Here's how the part is built. I have some questions about the finished solid (model axes, mm). A direction names the side the tool comes from. Round coordinates to 2 decimals unless told otherwise and drop trailing zeros. Order: outer loops, then holes, each group sorted by start corner. A loop starts at its lowest first (then second) coordinate and runs counter-clockwise, first axis right, second up.
```python
from build123d import *

# Parameters (mm, degrees)
SKETCH_1_R          = 14
EXTRUDE_1_DEPTH     = 5
SKETCH_2_R          = 14
EXTRUDE_2_DEPTH     = 5
SKETCH_4_R          = 3.8
EXTRUDE_3_DEPTH     = 25
FILLET_1_R          = 2
SKETCH_3_W          = 3.2
SKETCH_3_H          = 5.5
CUT_EXTRUDE_1_DEPTH = 5.5


with BuildPart() as part:
    # Эскиз1 → Бобышка-Вытянуть1 (new body)
    with BuildSketch(Plane(origin=(0, 0, 0), x_dir=(1, 0, 0), z_dir=(0, 1, 0))):
        with Locations(Location((0, 0, 0), (0, 0, 270))):
            Circle(SKETCH_1_R)
        with BuildLine():
            ThreePointArc((-7.383246629, 9.45979224), (-7.957471899, 8.982128978), (-8.500867665, 8.469666401))
            ThreePointArc((-8.500867665, 8.469666401), (-8.106391079, 5.595437755), (-10.933724873, 4.945064246))
            ThreePointArc((-10.933724873, 4.945064246), (-11.220194912, 4.255258645), (-11.463194733, 3.548966963))
            ThreePointArc((-11.463194733, 3.548966963), (-9.77818241, 1.187286301), (-11.979418514, -0.702518371))
            ThreePointArc((-11.979418514, -0.702518371), (-11.912506489, -1.446440163), (-11.799442035, -2.184758036))
            ThreePointArc((-11.799442035, -2.184758036), (-9.20990999, -3.492858137), (-10.280771741, -6.189162496))
            ThreePointArc((-10.280771741, -6.189162496), (-9.875806391, -6.816776961), (-9.432579364, -7.417981298))
            ThreePointArc((-9.432579364, -7.417981298), (-6.531758184, -7.372830869), (-6.226924059, -10.25794408))
            ThreePointArc((-6.226924059, -10.25794408), (-5.576678065, -10.625472308), (-4.904826437, -10.951834441))
            ThreePointArc((-4.904826437, -10.951834441), (-2.357259293, -9.563776902), (-0.746563118, -11.976754298))
            ThreePointArc((-0.746563118, -11.976754298), (0, -12), (0.746563118, -11.976754298))
            ThreePointArc((0.746563118, -11.976754298), (2.357259293, -9.563776902), (4.904826437, -10.951834441))
            ThreePointArc((4.904826437, -10.951834441), (5.576678065, -10.625472308), (6.226924059, -10.25794408))
            ThreePointArc((6.226924059, -10.25794408), (6.531758184, -7.372830869), (9.432579364, -7.417981298))
            ThreePointArc((9.432579364, -7.417981298), (9.875806391, -6.816776961), (10.280771741, -6.189162496))
            ThreePointArc((10.280771741, -6.189162496), (9.20990999, -3.492858137), (11.799442035, -2.184758036))
            ThreePointArc((11.799442035, -2.184758036), (11.912506489, -1.446440163), (11.979418514, -0.702518371))
            ThreePointArc((11.979418514, -0.702518371), (9.77818241, 1.187286301), (11.463194733, 3.548966963))
            ThreePointArc((11.463194733, 3.548966963), (11.220194912, 4.255258645), (10.933724873, 4.945064246))
            ThreePointArc((10.933724873, 4.945064246), (8.106391079, 5.595437755), (8.500867665, 8.469666401))
            ThreePointArc((8.500867665, 8.469666401), (7.957471899, 8.982128978), (7.383246629, 9.45979224))
            ThreePointArc((7.383246629, 9.45979224), (4.577523245, 8.721741853), (3.591094261, 11.450067336))
            ThreePointArc((3.591094261, 11.450067336), (2.871787971, 11.651301809), (2.14135556, 11.807395833))
            ThreePointArc((2.14135556, 11.807395833), (0, 9.85), (-2.14135556, 11.807395833))
            ThreePointArc((-2.14135556, 11.807395833), (-2.871787971, 11.651301809), (-3.591094261, 11.450067336))
            ThreePointArc((-3.591094261, 11.450067336), (-4.577523245, 8.721741853), (-7.383246629, 9.45979224))
        make_face(mode=Mode.SUBTRACT)
    extrude(amount=EXTRUDE_1_DEPTH)

    # Эскиз2 → Бобышка-Вытянуть2 (add)
    with BuildSketch(Plane(origin=(0, 5, 0), x_dir=(1, 0, 0), z_dir=(0, 1, 0))):
        with Locations(Location((0, 0, 0), (0, 0, 270))):
            Circle(SKETCH_2_R)
    extrude(amount=EXTRUDE_2_DEPTH)

    # Эскиз4 → Бобышка-Вытянуть3 (add)
    with BuildSketch(Plane.XZ.offset(-5)):
        with Locations(Location((0, 0, 0), (0, 0, 90))):
            Circle(SKETCH_4_R)
    extrude(amount=EXTRUDE_3_DEPTH)

    # Скругление1
    fillet_1_edges = [part.edges().sort_by_distance(p)[0] for p in [
        (0, -20, -3.8),
    ]]
    fillet(fillet_1_edges, radius=FILLET_1_R)

    # Эскиз3 → Вырез-Вытянуть1 (cut)
    with BuildSketch(Plane(origin=(0, 10, 0), x_dir=(1, 0, 0), z_dir=(0, 1, 0))):
        Rectangle(SKETCH_3_W, SKETCH_3_H)
    extrude(amount=-CUT_EXTRUDE_1_DEPTH, mode=Mode.SUBTRACT)


solid = part.part
```
1) We'd pull the mould along X, two halves only. Please class faces 1 (the cylindrical face through (-5.59, 2.46, 10.62)), 2 (the flat face through (0, 10, 3)): +X half, -X half, draft (parallel to the pull), parting line (faces both ways), or undercut.
2) I'm going to push flat-ended pins straight in: pin 1 (3 mm diameter, centred on y = 6, z = -0.5, fed in from -X); pin 2 (3 mm diameter, centred on y = -11, z = 1.5, fed in from -X); pin 3 (1 mm diameter, centred on x = -1.5, y = -7.5, fed in from -Z); pin 4 (1 mm diameter, centred on x = 4.5, y = 6.5, fed in from +Z). Where does each tip first touch, or does it pass through?
3) If we section it at A-A (y = 1.75): Write out the boundary of the cut face in (x, z), plus the area to 3 significant figures.
4) If we section it at C-C (z = 8): Write out the boundary of the cut face in (x, y), plus the area to 3 significant figures.
5) I need wall thicknesses on line 1 (Y direction, x = -0.5, z = -8); line 2 (Y direction, x = 11, z = -5.75); line 3 (Z direction, x = 2, y = -9.5). Which ranges of each line are inside material? Lowest first, please.
6) For faces 3 (the cylindrical face through (1.46, -6.34, 3.51)), 4 (the flat face through (0, 4.5, 0)), which set-ups out of +Z, -Z, +X, -X, +Y, -Y let a thin tool reach every point of the face, with its end or its side?
7) If we section it at B-B (z = -9): Write out the boundary of the cut face in (x, y).
Solutions:
1. face 1: undercut
1. face 2: draft
2. pin 1: stops at x = -14
2. pin 2: stops at x = -3.8
2. pin 3: stops at z = -3.67
2. pin 4: stops at z = 13.42
3. outline: circle Ø28 at (0, 0); circle Ø7.6 at (0, 0); hole (-11.98, 0.7) arc R2.15 cw to (-11.46, -3.55) arc R12 ccw to (-10.93, -4.95) arc R2.15 cw to (-8.5, -8.47) arc R12 ccw to (-7.38, -9.46) arc R2.15 cw to (-3.59, -11.45) arc R12 ccw to (-2.14, -11.81) arc R2.15 cw to (2.14, -11.81) arc R12 ccw to (3.59, -11.45) arc R2.15 cw to (7.38, -9.46) arc R12 ccw to (8.5, -8.47) arc R2.15 cw to (10.93, -4.95) arc R12 ccw to (11.46, -3.55) arc R2.15 cw to (11.98, 0.7) arc R12 ccw to (11.8, 2.18) arc R2.15 cw to (10.28, 6.19) arc R12 ccw to (9.43, 7.42) arc R2.15 cw to (6.23, 10.26) arc R12 ccw to (4.9, 10.95) arc R2.15 cw to (0.75, 11.98) arc R12 ccw to (-0.75, 11.98) arc R2.15 cw to (-4.9, 10.95) arc R12 ccw to (-6.23, 10.26) arc R2.15 cw to (-9.43, 7.42) arc R12 ccw to (-10.28, 6.19) arc R2.15 cw to (-11.8, 2.18) arc R12 ccw to start
3. area: 300 mm2
4. outline: (-11.49, 0) - (-6.04, 0) - (-6.04, 5) - (6.04, 5) - (6.04, 0) - (11.49, 0) - (11.49, 10) - (-11.49, 10) - close
4. area: 169 mm2
5. line 1: y = 5 to 10
5. line 2: y = 0 to 10
5. line 3: z = -3.23 to 3.23
6. face 3: -Y
6. face 4: +Y
7. outline: (-10.72, 0) - (-7.94, 0) - (-7.94, 5) - (-6.98, 5) - (-6.98, 0) - (-4.17, 0) - (-4.17, 5) - (4.17, 5) - (4.17, 0) - (6.98, 0) - (6.98, 5) - (7.94, 5) - (7.94, 0) - (10.72, 0) - (10.72, 10) - (-10.72, 10) - close
